```python
from build123d import *

# Parameters (mm, degrees)
BOSS_EXTRUDE1_DEPTH = 240


with BuildPart() as part:
    # Sketch1 → Boss-Extrude1 (new body)
    with BuildSketch(Plane.XY):
        with BuildLine():
            Line((-4.005405916, -48.006392066), (-5.596014404, -45.690783174))
            ThreePointArc((-5.596014404, -45.690783174), (-5.602314544, -45.474072701), (-5.407495225, -45.378948813))
            ThreePointArc((-5.407495225, -45.378948813), (-4.886118258, -45.438044064), (-4.364097153, -45.491149206))
            ThreePointArc((-4.364097153, -45.491149206), (-4.281696906, -45.51790434), (-4.218342055, -45.576995799))
            Line((-4.218342055, -45.576995799), (-3.016281965, -47.326955674))
            ThreePointArc((-3.016281965, -47.326955674), (-2.9606913, -48.824573862), (-4.291137006, -49.514403391))
            ThreePointArc((-4.291137006, -49.514403391), (-6.183725625, -49.313806762), (-8.067246452, -49.040896553))
            ThreePointArc((-8.067246452, -49.040896553), (-8.970999234, -48.484593683), (-9.22486491, -47.4541597))
            ThreePointArc((-9.22486491, -47.4541597), (-12.237087805, -44.938183329), (-13.103030303, -48.766207291))
            ThreePointArc((-13.103030303, -48.766207291), (0, -54.084716391), (13.103030303, -48.766207291))
            ThreePointArc((13.103030303, -48.766207291), (12.237087805, -44.938183329), (9.22486491, -47.4541597))
            ThreePointArc((9.22486491, -47.4541597), (8.970999234, -48.484593683), (8.067246452, -49.040896553))
            ThreePointArc((8.067246452, -49.040896553), (6.183725625, -49.313806762), (4.291137006, -49.514403391))
            ThreePointArc((4.291137006, -49.514403391), (2.9606913, -48.824573862), (3.016281965, -47.326955674))
            Line((3.016281965, -47.326955674), (4.218342055, -45.576995799))
            ThreePointArc((4.218342055, -45.576995799), (4.281696906, -45.51790434), (4.364097153, -45.491149206))
            ThreePointArc((4.364097153, -45.491149206), (4.886118258, -45.438044064), (5.407495225, -45.378948813))
            ThreePointArc((5.407495225, -45.378948813), (5.602314544, -45.474072701), (5.596014404, -45.690783174))
            Line((5.596014404, -45.690783174), (4.005405916, -48.006392066))
            ThreePointArc((4.005405916, -48.006392066), (3.997464392, -48.220337521), (4.187528064, -48.318884597))
            ThreePointArc((4.187528064, -48.318884597), (6.034420378, -48.123131348), (7.872463841, -47.856810519))
            ThreePointArc((7.872463841, -47.856810519), (8.001571382, -47.777338681), (8.037837907, -47.630133826))
            ThreePointArc((8.037837907, -47.630133826), (12.621655355, -43.801474132), (13.939393939, -49.626727987))
            ThreePointArc((13.939393939, -49.626727987), (0, -55.284716391), (-13.939393939, -49.626727987))
            ThreePointArc((-13.939393939, -49.626727987), (-12.621655355, -43.801474132), (-8.037837907, -47.630133826))
            ThreePointArc((-8.037837907, -47.630133826), (-8.001571382, -47.777338681), (-7.872463841, -47.856810519))
            ThreePointArc((-7.872463841, -47.856810519), (-6.034420378, -48.123131348), (-4.187528064, -48.318884597))
            ThreePointArc((-4.187528064, -48.318884597), (-3.997464392, -48.220337521), (-4.005405916, -48.006392066))
        make_face()
    extrude(amount=-BOSS_EXTRUDE1_DEPTH)


solid = part.part
```
The model under review builds one solid part; all positions refer to its coordinate system, in mm. A direction names the side the tool comes from. Give positions to 0.01 mm unless a question says otherwise; leave off trailing zeros. Write each loop counter-clockwise with the first axis right and the second up, starting at its lowest first coordinate (ties: lowest second). Pieces come first, ordered by that corner, then holes. Notation, with made-up numbers: (38.5, 80) - (50.5, 80) arc R31 ccw to (50.5, 114) - close; hole circle Ø7 at (28.5, 21.25). An arc over 180 degrees is marked (long way). Answer in a Markdown table with one row per item. Add a question column.
1. Wall thickness on line 1 along X through (y, z) = (-47.25, -64); line 2 along X through (y, z) = (-47.5, -133); line 3 along X through (y, z) = (-48.5, -51.5): over which ranges is each line inside the solid? List them lowest first. Write a range as [from, to].
2. We need section A-A on z = -146. Write out the cut boundary in (x, y).
3. Tool access review of faces 1 (the flat face through (-3.3, -48.6, -240)), 2 (the cylindrical face through (-6.157, -49.317, -118.32)): name each direction out of +Z, -Z, +X, -X, +Y, -Y from which nothing blocks a thin tool from reaching the whole face with its end or side.
4. Draft analysis for pull direction X (two halves, no side actions). For faces 3 (the cylindrical face through (12.3, -44.96, -118.32)), 4 (the cylindrical face through (0.216, -55.284, -118.32)), 5 (the flat face through (-3.3, -48.6, 0)), state which applies: +X half, -X half, draft (parallel to the pull), parting line (faces both ways), or undercut.
5. Insertion check: P1, Ø1.5, axis at y = -54, z = -142, coming from the -X side; P2, Ø12, axis at x = 6.5, z = -52, coming from the -Y side; P3, Ø1.5, axis at x = 5.5, z = -170, coming from the -Y side. Each pin has a flat end and moves straight along its axis. Give the tip position at first contact, or say it passes through.
Ans:
| question | item | result |
|---|---|---|
| 1 | line 1 | x = [-15, -13.8], [-9.2, -8], [-4.52, -3.07], [3.07, 4.52], [8, 9.2], [13.8, 15] |
| 1 | line 2 | x = [-14.98, -13.77], [-9.23, -8.02], [-4.35, -2.91], [2.91, 4.35], [8.02, 9.23], [13.77, 14.98] |
| 1 | line 3 | x = [-14.72, -13.34], [-8.96, -2.82], [2.82, 8.96], [13.34, 14.72] |
| 2 | outline | (-13.94, -49.63) arc R20 ccw to (13.94, -49.63) arc R3.5 ccw (long way) to (8.04, -47.63) arc R0.2 cw to (7.87, -47.86) arc R48.5 cw to (4.19, -48.32) arc R0.2 cw to (4.01, -48.01) - (5.6, -45.69) arc R0.2 ccw to (5.41, -45.38) arc R45.7 cw to (4.36, -45.49) arc R0.2 ccw to (4.22, -45.58) - (3.02, -47.33) arc R1.4 ccw to (4.29, -49.51) arc R49.7 ccw to (8.07, -49.04) arc R1.4 ccw to (9.22, -47.45) arc R2.3 cw (long way) to (13.1, -48.77) arc R18.8 cw to (-13.1, -48.77) arc R2.3 cw (long way) to (-9.22, -47.45) arc R1.4 ccw to (-8.07, -49.04) arc R49.7 ccw to (-4.29, -49.51) arc R1.4 ccw to (-3.02, -47.33) - (-4.22, -45.58) arc R0.2 ccw to (-4.36, -45.49) arc R45.7 cw to (-5.41, -45.38) arc R0.2 ccw to (-5.6, -45.69) - (-4.01, -48.01) arc R0.2 cw to (-4.19, -48.32) arc R48.5 cw to (-7.87, -47.86) arc R0.2 cw to (-8.04, -47.63) arc R3.5 ccw (long way) to start |
| 3 | face 1 | -Z, +X, -X, +Y, -Y |
| 3 | face 2 | +Z, -Z |
| 4 | face 3 | undercut |
| 4 | face 4 | parting line |
| 4 | face 5 | draft |
| 5 | P1 | stops at x = -8.79 |
| 5 | P2 | stops at y = -55.28 |
| 5 | P3 | stops at y = -54.71 |
